Build history of the part. All positions in model axes, mm. A direction names the side the tool comes from. Give positions to 0.01 mm unless a question says otherwise; leave off trailing zeros. Order: outer loops, then holes, each group sorted by start corner. A loop starts at its lowest first (then second) coordinate and runs counter-clockwise, first axis right, second up. Notation, with made-up numbers: M 76.5,-7 L 100.5,-7 A15 cw 100.5,3 Z; hole C 57.5,20 d9. An arc over 180 degrees is marked long. Use CSV: the item, a comma, the result in double quotes. Start each with the question number.
Item 1: Band-saw the part on B-B on y = -60. Write the cut outline in (x, z), plus the area to 3 significant figures.
Item 2: Pin check, flat tips, straight feed: P1, Ø3, axis at y = -18, z = -14.5, coming from the -X side; P2, Ø4, axis at y = -44.5, z = 19, coming from the -X side; P3, Ø3, axis at y = -26.5, z = 29.5, coming from the -X side; P4, Ø15, axis at x = -18, y = -35, coming from the -Z side. Stop position of each tip, or through.
Item 3: Two-plate mould, pull along Z, no slides. Class faces 5 (the flat face through (13.236, -37, 31)), 6 (the flat face through (1, -37, -10.823)), 7 (the flat face through (3, -37, 36.177)): pulls with the +Z half, pulls with the -Z half, needs draft (parallel to the pull), parting line crosses it, or undercut.
Item 4: Band-saw the part on A-A on x = 39. Write the cut outline in (y, z).
Item 5: Band-saw the part on D-D on x = 23. Write the cut outline in (y, z), plus the area to 3 significant figures.
Item 6: Band-saw the part on C-C on z = -18. Write the cut outline in (x, y).
Item 7: Which spindle directions (+Z, -Z, +X, -X, +Y, -Y) get a long thin tool onto all of the face, cutting with end or side? Do faces 1 (the flat face through (25, -37, 16.177)), 2 (the flat face through (-39, -37, 11.177)), 3 (the flat face through (1.01, -17.77, -19.95)), 4 (the flat face through (35.236, -37, 31)). Say none if no direction does.
Item 8: Wall check: line 1 along Z through (x, y) = (39, -17.5); line 2 along Z through (x, y) = (41.5, -38.5); line 3 along Z through (x, y) = (7, -19). Give the ranges that are in metal, low to high.
from build123d import *

# Parameters (mm, degrees)
F1_DEPTH = 75
F3_DEPTH = 110.001


with BuildPart() as f1:
    # F0 (on Front) → F1 (new body)
    with BuildSketch(Plane.XZ):
        Polygon((-54.763541, 11.177084), (-54.763541, -28.822916), (55.236459, -28.822916), (55.236459, 36.177084), (35.236459, 36.177084), (35.236459, 26.177084), (43.236459, 26.177084), (43.236459, 16.177084), (5.236459, 16.177084), (5.236459, 26.177084), (13.236459, 26.177084), (13.236459, 36.177084), (-6.763541, 36.177084), (-22.763541, 11.177084), align=None)
    extrude(amount=F1_DEPTH)

    # F2 (on face) → F3 (cut, through all)
    with BuildSketch(Plane.YZ.offset(55.236459)):
        Polygon((-12.5, -10.822916), (-62.5, -10.822916), (-52.107695, -28.822916), (-22.892305, -28.822916), align=None)
    extrude(amount=-F3_DEPTH, mode=Mode.SUBTRACT)


solid = f1.part
Model answer:
1,outline,"M -54.76,-28.82 L 55.24,-28.82 L 55.24,-15.15 L -54.76,-15.15 Z; M -54.76,-10.82 L 55.24,-10.82 L 55.24,36.18 L 35.24,36.18 L 35.24,26.18 L 43.24,26.18 L 43.24,16.18 L 5.24,16.18 L 5.24,26.18 L 13.24,26.18 L 13.24,36.18 L -6.76,36.18 L -22.76,11.18 L -54.76,11.18 Z"
1,area,"5,070 mm^2"
2,P1,"passes through"
2,P2,"stops at x = -19.04"
2,P3,"stops at x = -12"
2,P4,"stops at z = -10.82"
3,face 5,"needs draft"
3,face 6,"undercut"
3,face 7,"pulls with the +Z half"
4,outline,"M -75,-28.82 L -52.11,-28.82 L -62.5,-10.82 L -12.5,-10.82 L -22.89,-28.82 L 0,-28.82 L 0,16.18 L -75,16.18 Z; M -75,26.18 L 0,26.18 L 0,36.18 L -75,36.18 Z"
5,outline,"M -75,-28.82 L -52.11,-28.82 L -62.5,-10.82 L -12.5,-10.82 L -22.89,-28.82 L 0,-28.82 L 0,16.18 L -75,16.18 Z"
5,area,"2,660 mm^2"
6,outline,"M -54.76,-75 L 55.24,-75 L 55.24,-58.36 L -54.76,-58.36 Z; M -54.76,-16.64 L 55.24,-16.64 L 55.24,0 L -54.76,0 Z"
7,face 1,"+Y, -Y"
7,face 2,"+Z, -X, +Y, -Y"
7,face 3,"+X, -X"
7,face 4,"+Z, +Y, -Y"
8,line 1,"z = -28.82 to -19.48, -10.82 to 16.18, 26.18 to 36.18"
8,line 2,"z = -10.82 to 16.18, 26.18 to 36.18"
8,line 3,"z = -28.82 to -22.08, -10.82 to 16.18, 26.18 to 36.18"
